from build123d import *

# Parameters (mm, degrees)
SKETCH1_R           = 2.159
BOSS_EXTRUDE1_DEPTH = 5.8928


with BuildPart() as part:
    # Sketch1 → Boss-Extrude1 (new body)
    # profile 1 of 3: a face of its own
    with BuildSketch(Plane(origin=(0, 0, 0), x_dir=(1, 0, 0), z_dir=(0, 1, 0))):
        with BuildLine():
            Line((22.86, -56.388), (25.4, -56.388))
            Line((25.4, -56.388), (27.94, -56.388))
            Line((27.94, -56.388), (27.94, -57.404))
            Line((27.94, -57.404), (30.1625, -57.404))
            Line((30.1625, -57.404), (30.1625, -60.452))
            Line((30.1625, -60.452), (27.94, -60.452))
            Line((27.94, -60.452), (27.94, -63.5))
            Line((27.94, -63.5), (99.06, -63.5))
            Line((99.06, -63.5), (99.06, -60.452))
            Line((99.06, -60.452), (96.8375, -60.452))
            Line((96.8375, -60.452), (96.8375, -57.404))
            Line((96.8375, -57.404), (99.06, -57.404))
            Line((99.06, -57.404), (99.06, -56.388))
            Line((99.06, -56.388), (101.6, -56.388))
            Line((101.6, -56.388), (104.14, -56.388))
            Line((104.14, -56.388), (104.14, -57.404))
            Line((104.14, -57.404), (106.3625, -57.404))
            Line((106.3625, -57.404), (106.3625, -60.452))
            Line((106.3625, -60.452), (104.14, -60.452))
            Line((104.14, -60.452), (104.14, -63.5))
            Line((104.14, -63.5), (175.26, -63.5))
            Line((175.26, -63.5), (175.26, -60.452))
            Line((175.26, -60.452), (173.0375, -60.452))
            Line((173.0375, -60.452), (173.0375, -57.404))
            Line((173.0375, -57.404), (175.26, -57.404))
            Line((175.26, -57.404), (175.26, -56.388))
            Line((175.26, -56.388), (177.8, -56.388))
            Line((177.8, -56.388), (180.34, -56.388))
            Line((180.34, -56.388), (180.34, -57.404))
            Line((180.34, -57.404), (182.5625, -57.404))
            Line((182.5625, -57.404), (182.5625, -60.452))
            Line((182.5625, -60.452), (180.34, -60.452))
            Line((180.34, -60.452), (180.34, -63.5))
            Line((180.34, -63.5), (251.46, -63.5))
            Line((251.46, -63.5), (251.46, -60.452))
            Line((251.46, -60.452), (249.2375, -60.452))
            Line((249.2375, -60.452), (249.2375, -57.404))
            Line((249.2375, -57.404), (251.46, -57.404))
            Line((251.46, -57.404), (251.46, -56.388))
            Line((251.46, -56.388), (254, -56.388))
            Line((254, -56.388), (256.54, -56.388))
            Line((256.54, -56.388), (256.54, -57.404))
            Line((256.54, -57.404), (258.7625, -57.404))
            Line((258.7625, -57.404), (258.7625, -60.452))
            Line((258.7625, -60.452), (256.54, -60.452))
            Line((256.54, -60.452), (256.54, -63.5))
            Line((256.54, -63.5), (279.4, -63.5))
            Line((279.4, -63.5), (279.4, -31.75))
            add(Edge.make_bspline(
                [(268.339603776, 0), (275.019525549, -6.158991848), (279.385214725, -16.365397032), (279.4, -31.75)],
                knots=[0.805473307, 0.805473307, 0.805473307, 0.805473307, 1, 1, 1, 1], degree=3))
            Line((268.339603776, 0), (232.176763275, 0))
            Line((232.176763275, 0), (229.641134322, -14.380266384))
            Line((229.641134322, -14.380266384), (223.837859195, -13.356992403))
            Line((223.837859195, -13.356992403), (226.078012822, -0.652449861))
            Line((226.078012822, -0.652449861), (220.106261854, -0.652449861))
            add(Edge.make_bspline(
                [(167.647045609, -36.208320755), (182.540854706, -36.177050532), (193.471525933, -31.320671219), (205.978352833, -11.056890294), (216.80246247, -2.714612362), (220.106261854, -0.652449861)],
                knots=[0, 0, 0, 0, 0.18449289, 0.370391028, 0.445681017, 0.445681017, 0.445681017, 0.445681017], degree=3))
            Line((167.647045609, -36.208320755), (40.664262654, -36.208320755))
            add(Edge.make_bspline(
                [(40.664262654, -36.208320755), (0, -36.208320755), (0, -63.5)],
                knots=[1.570796327, 1.570796327, 1.570796327, 3.141592654, 3.141592654, 3.141592654], degree=2, weights=[1, 0.707106781, 1]))
            Line((0, -63.5), (22.86, -63.5))
            Line((22.86, -63.5), (22.86, -60.452))
            Line((22.86, -60.452), (20.6375, -60.452))
            Line((20.6375, -60.452), (20.6375, -57.404))
            Line((20.6375, -57.404), (22.86, -57.404))
            Line((22.86, -57.404), (22.86, -56.388))
        make_face()
        with Locations(Location((221.854115864, -41.575001242, 0), (0, 0, 270))):
            Circle(SKETCH1_R, mode=Mode.SUBTRACT)
        Polygon((221.76484725, -25.113627358), (227.568122377, -26.13690134), (225.7922594, -36.208320755), (219.988984273, -35.185046774), align=None, mode=Mode.SUBTRACT)
        with Locations(Location((225.702990786, -19.746946871, 0), (0, 0, 270))):
            Circle(SKETCH1_R, mode=Mode.SUBTRACT)
    # profile 2 of 3: a face of its own
    with BuildSketch(Plane(origin=(0, 0, 0), x_dir=(1, 0, 0), z_dir=(0, 1, 0))):
        with BuildLine():
            Line((233.123919707, 5.371591052), (232.176763275, 0))
            Line((232.176763275, 0), (268.339603776, 0))
            add(Edge.make_bspline(
                [(264.58250195, 2.898755616), (265.899962004, 2.055359977), (267.156104906, 1.091204379), (268.339603776, 0)],
                knots=[0.771008514, 0.771008514, 0.771008514, 0.771008514, 0.805473307, 0.805473307, 0.805473307, 0.805473307], degree=3))
            add(Edge.make_bspline(
                [(233.123919707, 5.371591052), (239.398286694, 7.344939742), (250.719959286, 8.655748308), (260.759413307, 5.346174252), (264.58250195, 2.898755616)],
                knots=[0.539626218, 0.539626218, 0.539626218, 0.539626218, 0.670996405, 0.771008514, 0.771008514, 0.771008514, 0.771008514], degree=3))
        make_face()
    # profile 3 of 3: a face of its own
    with BuildSketch(Plane(origin=(0, 0, 0), x_dir=(1, 0, 0), z_dir=(0, 1, 0))):
        with BuildLine():
            Line((235.922949985, 21.245680584), (233.123919707, 5.371591052))
            add(Edge.make_bspline(
                [(233.123919707, 5.371591052), (239.398286694, 7.344939742), (250.719959286, 8.655748308), (260.759413307, 5.346174252), (264.58250195, 2.898755616)],
                knots=[0.539626218, 0.539626218, 0.539626218, 0.539626218, 0.670996405, 0.771008514, 0.771008514, 0.771008514, 0.771008514], degree=3))
            Line((264.58250195, 2.898755616), (235.922949985, 21.245680584))
        make_face()
    extrude(amount=BOSS_EXTRUDE1_DEPTH)


solid = part.part
Input: part model. Units: mm. Frame: model coordinates. A direction names the side the tool comes from. Give positions to 0.01 mm unless a question says otherwise; leave off trailing zeros. Order: outer loops, then holes, each group sorted by start corner. A loop starts at its lowest first (then second) coordinate and runs counter-clockwise, first axis right, second up.
Q1. Section C-C on z = -14.5. Output: boundary loops of the cut face in (x, y), and give its area (3 significant figures).
Checked values:
outline: (234.73, 0) - (246.46, 0) - (246.46, 5.89) - (234.73, 5.89) - close
area: 69.1 mm2
Q2. Draft query along Z for faces 5 (the flat face through (220.864, 2.905, 30.22)), 6 (the flat face through (63, 3, 63.5)), 7 (the flat face through (223, 3, 0.652)), 8 (the flat face through (224.63, 2.91, 25.62)). Return one class per face: +Z half, -Z half, draft (parallel to the pull), parting line (faces both ways), or undercut.
Checked values:
face 5: undercut
face 6: +Z half
face 7: -Z half
face 8: undercut
Q3. Section B-B on y = 3.55. State how many separate pieces and enclosed holes the cut face has, and give its area (3 significant figures).
Checked values:
separate pieces: 1
enclosed holes: 3
area: 10,100 mm2
Q4. Section A-A on x = 163. Output: boundary loops of the cut face in (y, z), and give its area (3 significant figures).
Checked values:
outline: (0, 36.21) - (5.89, 36.21) - (5.89, 63.5) - (0, 63.5) - close
area: 161 mm2
Q5. Ray query, probe 1 along X at (y, z) = (3.1, 56.5); probe 2 along Z at (x, y) = (100, 5.5); probe 3 along X at (y, z) = (4.65, 1.5) (3 decimals). Return the intervals inside material, ascending.
Checked values:
probe 1: x = 1.36 to 22.86, 27.94 to 99.06, 104.14 to 175.26, 180.34 to 251.46, 256.54 to 279.4
probe 2: z = 36.21 to 56.39
probe 3: x = 218.788 to 225.929, 231.912 to 269.845
Q6. Contact query for flat-ended pins moving along their axis: pin 1 Ø2.5 at (y, z) = (3, 59) entering from -X; pin 2 Ø0.5 at (y, z) = (2, 57) entering from -X; pin 3 Ø1.1 at (y, z) = (4.5, 57) entering from -X. Output: stop coordinate, or through.
Checked values:
pin 1: stops at x = 0.29
pin 2: stops at x = 1.08
pin 3: stops at x = 0.98
Q7. Set-up query: faces 1 (the flat face through (250.453, 2.905, -11.944)), 2 (the flat face through (254, 3, 56.388)), 3 (the flat face through (105, 3, 36.208)), 4 (the flat face through (226.693, 2.905, 31.102)). Return all of +Z, -Z, +X, -X, +Y, -Y with unobstructed straight access to the full face (end or side cutting, diameter ignored); none if empty.
Checked values:
face 1: -Z, +X, +Y, -Y
face 2: +Z, +Y, -Y
face 3: -Z, -X, +Y, -Y
face 4: +Y, -Y
